Work out the finished part from the listing and answer in its coordinate system (mm). Face numbers are marked on the shaded views. A direction names the side the tool comes from. Round coordinates to 2 decimals unless told otherwise and drop trailing zeros. Loops run counter-clockwise (first coordinate to the right, second up) from the corner with the lowest first, then second, coordinate; pieces in that order, holes last.
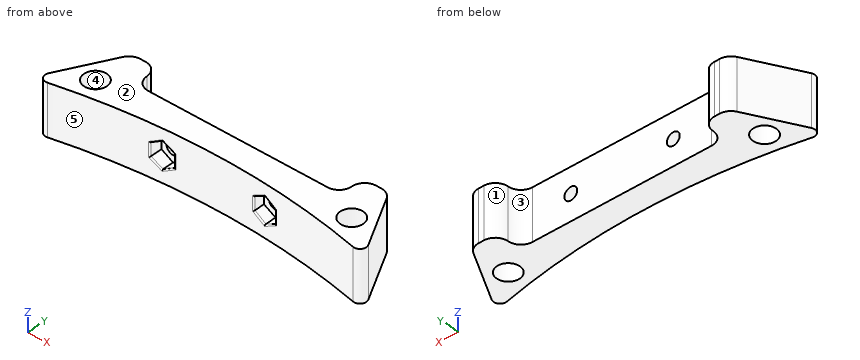
```python
from build123d import *

# Parameters (mm, degrees)
F0_R     = 4.5
F1_DEPTH = 20
F2_R     = 4.99999
F3_R     = 2.5
F4_R     = 2.5
F5_DEPTH = 25
F8_DEPTH = 6
F9_R     = 0.5


# Not quite as in the source:
# - a fillet or chamfer is up to 0.001 mm smaller than in the source, because OpenCascade refuses the exact size
# - a feature names something its author has since deleted; it is built from what else it names


with BuildPart() as f1:
    # F0 (on Top) → F1 (new body)
    with BuildSketch(Plane.XY):
        with BuildLine():
            Line((40, 0), (-40, 0))
            Line((-40, 0), (-40, 10))
            Line((-40, 10), (-50, 10))
            Line((-50, 10), (-65, -17.7922156823))
            ThreePointArc((-65, -17.7922156823), (0, -10), (65, -17.7922156823))
            Line((65, -17.7922156823), (50, 10))
            Line((50, 10), (40, 10))
            Line((40, 10), (40, 0))
        make_face()
        with Locations((-50, -6.2922156823)):
            Circle(F0_R, mode=Mode.SUBTRACT)
        with Locations((50, -6.2922156823)):
            Circle(F0_R, mode=Mode.SUBTRACT)
    extrude(amount=F1_DEPTH)

    # F2 (radius 5 in the source; OpenCascade refuses exactly that, so slightly less here)
    f2_edges = [f1.edges().sort_by_distance(p)[0] for p in [
        (-40, 10, 10),
        (-40, 0, 10),
        (40, 10, 10),
        (40, 0, 10),
        (-50, 10, 10),
        (50, 10, 10),
    ]]
    fillet(f2_edges, radius=F2_R)

    # F3
    f3_edges = [f1.edges().sort_by_distance(p)[0] for p in [
        (-65, -17.792216, 10),
        (65, -17.792216, 10),
    ]]
    fillet(f3_edges, radius=F3_R)

    # F4 (on face) → F5 (cut)
    with BuildSketch(Plane(origin=(0, 0, 0), x_dir=(-1, 0, 0), z_dir=(0, 1, 0))):
        with Locations((-19.9995623863, 10.1323040371)):
            Circle(F4_R)
        with Locations((20, 10)):
            Circle(F4_R)
    extrude(amount=-F5_DEPTH, mode=Mode.SUBTRACT)

    # F7 (on offset) → F8 (cut)
    with BuildSketch(Plane.XZ.offset(12)):
        Polygon((-15.5, 7.4019237886), (-15.5, 12.5980762114), (-20, 15.1961524227), (-24.5, 12.5980762114), (-24.5, 7.4019237886), (-20, 4.8038475773), align=None)
        Polygon((15.5, 12.5980762114), (15.5, 7.4019237886), (20, 4.8038475773), (24.5, 7.4019237886), (24.5, 12.5980762114), (20, 15.1961524227), align=None)
    extrude(amount=-F8_DEPTH, mode=Mode.SUBTRACT)

    # F9
    f9_edges = [f1.edges().sort_by_distance(p)[0] for p in [
        (-22.250563, -10.901637, 13.896789),
        (-24.5, -11.093538, 10),
        (-22.250563, -10.901637, 6.103211),
        (-17.750448, -10.573468, 6.102627),
        (-15.5, -10.437166, 10),
        (-17.750448, -10.573468, 13.897373),
        (17.750448, -10.573468, 13.897373),
        (15.5, -10.437166, 10),
        (17.750448, -10.573468, 6.102627),
        (22.250563, -10.901637, 6.103211),
        (24.5, -11.093538, 10),
        (22.250563, -10.901637, 13.896789),
    ]]
    fillet(f9_edges, radius=F9_R)


solid = f1.part
```
1. Find section A-A (x = -49.5). Write down the section's boundary in (y, z), then the cut area to 3 significant figures.
Answer key:
outline: (-14.49, 0) - (-10.76, 0) - (-10.76, 20) - (-14.49, 20) - close; (-1.82, 0) - (9.34, 0) - (9.34, 20) - (-1.82, 20) - close
area: 298 mm2
2. Determine the mould class of the marked faces 3, 4 and 5 for opening direction Y: +Y half, -Y half, draft (parallel to the pull), parting line (faces both ways), or undercut.
Answer key:
face 3: +Y half
face 4: undercut
face 5: -Y half
3. Given pin 1 (3 mm diameter, centred on y = 6, z = 12, fed in from -X); pin 2 (1.5 mm diameter, centred on x = 13, y = 2, fed in from +Z); pin 3 (10 mm diameter, centred on x = -21.5, z = 12, fed in from -Y); pin 4 (2.5 mm diameter, centred on y = -9, z = 9, fed in from -X), each flat-ended and moving along its own axis, determine where each tip first touches the part or whether it passes through.
Answer key:
pin 1: stops at x = -52.97
pin 2: passes through
pin 3: stops at y = -11.28
pin 4: stops at x = -60.93
4. Consider probe 1 along X at (y, z) = (-6.5, 18.5); probe 2 along Z at (x, y) = (-20, -2.75); probe 3 along Y at (x, z) = (50, 9). Determine where each line is inside the solid, lowest interval first.
Answer key:
probe 1: x = -58.91 to -54.5, -45.5 to 45.5, 54.5 to 58.91
probe 2: z = 0 to 7.5, 12.5 to 20
probe 3: y = -14.58 to -10.79, -1.79 to 9.01
5. Find section B-B (x = 43). Write down the section's boundary in (y, z), then the cut area to 3 significant figures.
Answer key:
outline: (-13.38, 0) - (9.58, 0) - (9.58, 20) - (-13.38, 20) - close
area: 459 mm2
6. Find section C-C (x = -30). Write down the section's boundary in (y, z), then the cut area to 3 significant figures.
Answer key:
outline: (-11.64, 0) - (0, 0) - (0, 20) - (-11.64, 20) - close
area: 233 mm2
7. Which of the six approach directions +Z, -Z, +X, -X, +Y, -Y give full straight-line access (tool end or side, diameter ignored) to the marked faces 1 and 2?
Answer key:
face 1: +Z, -Z, +Y
face 2: +Z, +X, -X, +Y, -Y
